```python
from build123d import *

# Parameters (mm, degrees)
F0_R     = 4.7625
F1_DEPTH = 50.8
F2_R     = 12.7


with BuildPart() as f1:
    # F0 (on Front) → F1 (new body)
    with BuildSketch(Plane.XZ):
        with BuildLine():
            ThreePointArc((171.7572451724, -35.3274357641), (173.9798664945, -16.0360244509), (174.7221865654, 3.3688088879))
            ThreePointArc((174.7221865654, 3.3688088879), (173.9798657597, 22.7736518176), (171.7572422416, 42.0650725533))
            ThreePointArc((171.7572422416, 42.0650725533), (155.3875841422, 100.5704095954), (125.5931558219, 153.5150241446))
            ThreePointArc((125.5931558219, 153.5150241446), (100.3273021851, 182.9739381109), (70.8683863051, 208.2397895165))
            ThreePointArc((70.8683863051, 208.2397895165), (17.9237694993, 238.0342138268), (-40.5815687826, 254.4038674949))
            ThreePointArc((-40.5815687826, 254.4038674949), (-79.2778230536, 257.3688088879), (-117.9740771, 254.4038645641))
            ThreePointArc((-117.9740771, 254.4038645641), (-176.4794141421, 238.0342064647), (-229.4240286913, 208.2397781444))
            ThreePointArc((-229.4240286913, 208.2397781444), (-258.8829426576, 182.9739245076), (-284.1487940632, 153.5150086276))
            ThreePointArc((-284.1487940632, 153.5150086276), (-313.9432183735, 100.5703918218), (-330.3128720416, 42.0650535399))
            ThreePointArc((-330.3128720416, 42.0650535399), (-333.2778134346, 3.3687992689), (-330.3128691108, -35.3274547775))
            ThreePointArc((-330.3128691108, -35.3274547775), (-313.9432110114, -93.8327918196), (-284.1487826911, -146.7774063688))
            ThreePointArc((-284.1487826911, -146.7774063688), (-258.8829290543, -176.2363203351), (-229.4240131743, -201.5021717407))
            ThreePointArc((-229.4240131743, -201.5021717407), (-176.4793963685, -231.296596051), (-117.9740580866, -247.6662497191))
            ThreePointArc((-117.9740580866, -247.6662497191), (-79.2778038156, -250.6311911121), (-40.5815497692, -247.6662467883))
            ThreePointArc((-40.5815497692, -247.6662467883), (17.9237872729, -231.2965886889), (70.8684018221, -201.5021603686))
            ThreePointArc((70.8684018221, -201.5021603686), (100.3273157884, -176.2363067318), (125.593167194, -146.7773908518))
            ThreePointArc((125.593167194, -146.7773908518), (155.3875915043, -93.832774046), (171.7572451724, -35.3274357641))
        make_face()
        with BuildLine():
            Line((-199.111355404, -160.7353111672), (-96.7847279201, -23.11836622))
            ThreePointArc((-96.7847279201, -23.11836622), (-91.4280109116, -25.9643668909), (-85.6278134346, -27.7397108454))
            Line((-85.6278134346, -27.7397108454), (-110.5818240092, -197.4054397645))
            ThreePointArc((-110.5818240092, -197.4054397645), (-157.0390796928, -184.3635151001), (-199.111355404, -160.7353111672))
        make_face(mode=Mode.SUBTRACT)
        with BuildLine():
            ThreePointArc((-243.3819243, -116.4647456663), (-267.0101314592, -74.3924717671), (-280.0520596864, -27.9352170836))
            Line((-280.0520596864, -27.9352170836), (-110.3863325182, -2.981194295))
            ThreePointArc((-110.3863325182, -2.981194295), (-108.6109879703, -8.7813915903), (-105.7649867513, -14.1381083077))
            Line((-105.7649867513, -14.1381083077), (-243.3819243, -116.4647456663))
        make_face(mode=Mode.SUBTRACT)
        with BuildLine():
            Line((-47.9737874631, -197.4054373639), (-72.9278102517, -27.7397101957))
            ThreePointArc((-72.9278102517, -27.7397101957), (-67.1276129564, -25.9643656478), (-61.770896239, -23.1183644288))
            Line((-61.770896239, -23.1183644288), (40.5557411196, -160.7353019775))
            ThreePointArc((40.5557411196, -160.7353019775), (-1.5165327796, -184.3635091367), (-47.9737874631, -197.4054373639))
        make_face(mode=Mode.SUBTRACT)
        with BuildLine():
            Line((84.8263066205, -116.4647330815), (-52.7906383267, -14.1381055976))
            ThreePointArc((-52.7906383267, -14.1381055976), (-49.9446376558, -8.7813885891), (-48.1692937013, -2.9811911121))
            Line((-48.1692937013, -2.9811911121), (121.4964352178, -27.9352016867))
            ThreePointArc((121.4964352178, -27.9352016867), (108.4545105534, -74.3924573703), (84.8263066205, -116.4647330815))
        make_face(mode=Mode.SUBTRACT)
        with BuildLine():
            Line((-243.3819334897, 123.2023508573), (-105.7649885425, 20.8757233734))
            ThreePointArc((-105.7649885425, 20.8757233734), (-108.6109892134, 15.5190063649), (-110.3863331679, 9.7188088879))
            Line((-110.3863331679, 9.7188088879), (-280.052062087, 34.6728194624))
            ThreePointArc((-280.052062087, 34.6728194624), (-267.0101374226, 81.1300751461), (-243.3819334897, 123.2023508573))
        make_face(mode=Mode.SUBTRACT)
        with BuildLine():
            Line((-110.5818394061, 204.1430551397), (-85.6278166175, 34.4773279715))
            ThreePointArc((-85.6278166175, 34.4773279715), (-91.4280139128, 32.7019834236), (-96.7847306302, 29.8559822046))
            Line((-96.7847306302, 29.8559822046), (-199.1113679888, 167.4729197533))
            ThreePointArc((-199.1113679888, 167.4729197533), (-157.0390940896, 191.1011269125), (-110.5818394061, 204.1430551397))
        make_face(mode=Mode.SUBTRACT)
        with Locations((-79.2778134346, 3.3688088879)):
            Circle(F0_R, mode=Mode.SUBTRACT)
        with BuildLine():
            Line((121.4964328172, 34.6728348594), (-48.169294351, 9.7188120708))
            ThreePointArc((-48.169294351, 9.7188120708), (-49.9446388989, 15.5190093661), (-52.7906401179, 20.8757260835))
            Line((-52.7906401179, 20.8757260835), (84.8262974308, 123.2023634421))
            ThreePointArc((84.8262974308, 123.2023634421), (108.45450459, 81.1300895429), (121.4964328172, 34.6728348594))
        make_face(mode=Mode.SUBTRACT)
        with BuildLine():
            ThreePointArc((-61.7708989491, 29.8559839958), (-67.1276159576, 32.7019846667), (-72.9278134346, 34.4773286212))
            Line((-72.9278134346, 34.4773286212), (-47.9738028601, 204.1430575403))
            ThreePointArc((-47.9738028601, 204.1430575403), (-1.5165471764, 191.1011328759), (40.5557285348, 167.472928943))
            Line((40.5557285348, 167.472928943), (-61.7708989491, 29.8559839958))
        make_face(mode=Mode.SUBTRACT)
    extrude(amount=F1_DEPTH)

    # F2
    f2_edges = [f1.edges().sort_by_distance(p)[0] for p in [
        (-229.424029, -50.8, 208.239778),
        (-229.424029, 0, 208.239778),
    ]]
    fillet(f2_edges, radius=F2_R)


solid = f1.part
```
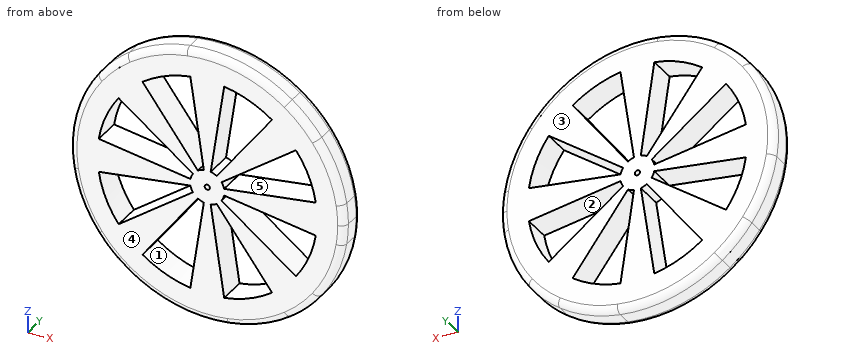
Build history of the part. All positions in model axes, mm. Face numbers are marked on the shaded views. A direction names the side the tool comes from. Coordinates: 2 decimals unless noted, no trailing zeros.
1. 3-axis set-ups, long thin cutter, end or side, ignore diameter. For the marked faces 4 and 5: which of +Z, -Z, +X, -X, +Y, -Y reach the whole face in a straight line?
Answer block:
face 4: +Z, -Z, +X, -X, -Y
face 5: +Y, -Y
2. Band-saw the part on A-A, the plane y = -25. Give the number of separate pieces and of enclosed holes in the cut face, and give its area (3 significant figures).
Answer block:
separate pieces: 1
enclosed holes: 9
area: 128,000 mm2
3. Drop flat-ended pins along their axis: pin 1 (10 mm diameter, centred on y = -13.5, z = -74.5, fed in from -X); pin 2 (2 mm diameter, centred on y = -35, z = -146.5, fed in from -X); pin 3 (4 mm diameter, centred on x = -88, y = -5.5, fed in from +Z). Give the stop position or say it passes through.
Answer block:
pin 1: stops at x = -322.6
pin 2: stops at x = -285.08
pin 3: stops at z = 256.11
4. Pull direction X, two halves, no side cores. Call the marked faces 1, 2 and 3: released by +X, released by -X, zero draft, split by the parting line, or undercut.
Answer block:
face 1: undercut
face 2: undercut
face 3: zero draft
5. Drill centre lines: probe 1 along X at (y, z) = (-37.5, -131); probe 2 along Z at (x, y) = (-207.5, -20); probe 3 along X at (y, z) = (-23.5, -60). Where is each one in solid material? Low to high.
Answer block:
probe 1: x = -294.83 to -177, -100.82 to -57.74, 18.45 to 136.27
probe 2: z = -215.89 to -89.78, -17.26 to 24, 96.52 to 222.63
probe 3: x = -325.25 to -272.34, -167.44 to -124.21, -90.37 to -68.18, -34.35 to 8.89, 113.79 to 166.69
